Work out the finished part from the listing and answer in its coordinate system (mm). Face numbers are marked on the shaded views. A direction names the side the tool comes from. Round coordinates to 2 decimals unless told otherwise and drop trailing zeros. Loops run counter-clockwise (first coordinate to the right, second up) from the corner with the lowest first, then second, coordinate; pieces in that order, holes last. Notation, with made-up numbers: (-5.5, 17) -> (4.5, 17) arc R25 ccw to (4.5, 49) -> close; hole circle Ø1 at (25, 83). An arc over 180 degrees is marked (long way). Use one line per item in the form item = value.
```python
from build123d import *

# Parameters (mm, degrees)
F1_DEPTH = 63.5
F0_W     = 25.4
F0_H     = 19.05
F2_DEPTH = 25.4
F3_DEPTH = 7.9375
F4_DEPTH = 25.4
F5_DEPTH = 63.5
F7_R     = 6.35


with BuildPart() as f1:
    # F0 (on Front) → F1 (new body)
    with BuildSketch(Plane.XZ):
        Polygon((-41.275, 9.525), (-41.275, -9.525), (41.275, -9.525), (41.275, 9.525), (22.225, 9.525), align=None)
    extrude(amount=F1_DEPTH)

    # F0 (on Front) → F2 (join)
    with BuildSketch(Plane.XZ):
        with Locations((73.025, 52.4002)):
            Rectangle(F0_W, F0_H)
        with BuildLine():
            Line((22.225, 9.525), (41.275, 9.525))
            Line((41.275, 9.525), (41.275, 27.0002))
            ThreePointArc((41.275, 27.0002), (45.9246798487, 38.2255201513), (57.15, 42.8752))
            Line((57.15, 42.8752), (60.325, 42.8752))
            Line((60.325, 42.8752), (60.325, 61.9252))
            Line((60.325, 61.9252), (57.15, 61.9252))
            add(Edge.make_bspline(
                [(52.9823235554, 61.6756394068), (54.3561666256, 61.7778957216), (55.7451531138, 61.8610815688), (57.15, 61.9252)],
                knots=[107.6072789541, 107.6072789541, 107.6072789541, 107.6072789541, 111.5045361635, 111.5045361635, 111.5045361635, 111.5045361635], degree=3))
            ThreePointArc((52.9823235554, 61.6756394068), (31.0223161682, 50.1756128892), (22.225, 27.0002))
            Line((22.225, 27.0002), (22.225, 9.525))
        make_face()
    extrude(amount=F2_DEPTH)

    # F0 (on Front) → F3 (join, symmetric)
    with BuildSketch(Plane.XZ):
        with BuildLine():
            add(Edge.make_bspline(
                [(-41.275, 9.525), (-11.3392454838, 41.4901042483), (15.0491037151, 58.8522374069), (52.9823235554, 61.6756394068)],
                knots=[0, 0, 0, 0, 107.6072789541, 107.6072789541, 107.6072789541, 107.6072789541], degree=3))
            Line((-41.275, 9.525), (22.225, 9.525))
            Line((22.225, 9.525), (22.225, 27.0002))
            ThreePointArc((22.225, 27.0002), (31.0223161682, 50.1756128892), (52.9823235554, 61.6756394068))
        make_face()
    extrude(amount=F3_DEPTH, both=True)

    # F0 (on Front) → F4 (join, symmetric)
    with BuildSketch(Plane.XZ):
        with BuildLine():
            Line((22.225, 9.525), (41.275, 9.525))
            Line((41.275, 9.525), (41.275, 27.0002))
            ThreePointArc((41.275, 27.0002), (45.9246798487, 38.2255201513), (57.15, 42.8752))
            Line((57.15, 42.8752), (60.325, 42.8752))
            Line((60.325, 42.8752), (60.325, 61.9252))
            Line((60.325, 61.9252), (57.15, 61.9252))
            add(Edge.make_bspline(
                [(52.9823235554, 61.6756394068), (54.3561666256, 61.7778957216), (55.7451531138, 61.8610815688), (57.15, 61.9252)],
                knots=[107.6072789541, 107.6072789541, 107.6072789541, 107.6072789541, 111.5045361635, 111.5045361635, 111.5045361635, 111.5045361635], degree=3))
            ThreePointArc((52.9823235554, 61.6756394068), (31.0223161682, 50.1756128892), (22.225, 27.0002))
            Line((22.225, 27.0002), (22.225, 9.525))
        make_face()
        with Locations((73.025, 52.4002)):
            Rectangle(F0_W, F0_H)
    extrude(amount=F4_DEPTH, both=True)

    # F0 (on Front) → F5 (join)
    with BuildSketch(Plane.XZ):
        Polygon((-41.275, 9.525), (-41.275, -9.525), (41.275, -9.525), (41.275, 9.525), (22.225, 9.525), align=None)
    extrude(amount=-F5_DEPTH)

    # F0 (on Front) → F6 (revolve)
    with BuildSketch(Plane.XZ):
        Polygon((85.725, 66.675), (85.725, 61.9252), (85.725, 42.8752), (85.725, 38.1), (111.125, 38.1), (111.125, 66.675), align=None)
    revolve(axis=Axis((85.725, 0, 52.3875), (0, 0, 1)))

    # F7
    f7_edges = [f1.edges().sort_by_distance(p)[0] for p in [
        (-41.275, -63.5, 0),
        (41.275, -63.5, 0),
        (41.275, 63.5, 0),
        (-41.275, 63.5, 0),
    ]]
    fillet(f7_edges, radius=F7_R)


solid = f1.part
```
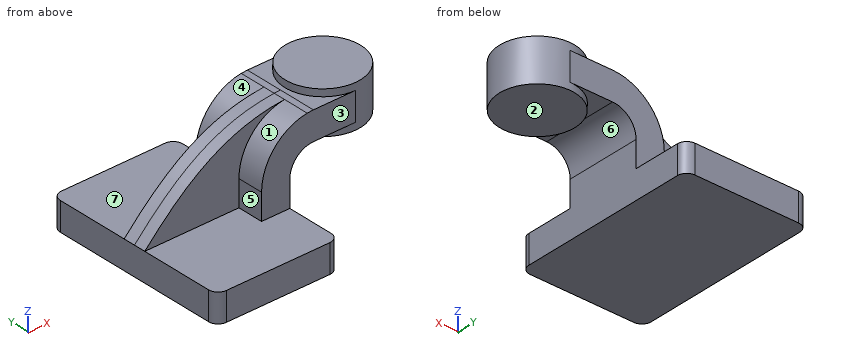
(1) Find section A-A, the plane z = 5. Write down the section's boundary in (x, y) (3 decimals), then the cut area to 3 significant figures.
Completed:
outline = (-41.275, -57.15) arc R6.35 ccw to (-34.925, -63.5) -> (34.925, -63.5) arc R6.35 ccw to (41.275, -57.15) -> (41.275, 57.15) arc R6.35 ccw to (34.925, 63.5) -> (-34.925, 63.5) arc R6.35 ccw to (-41.275, 57.15) -> close
area = 10,400 mm2
(2) Find section B-B, the plane y = -28. Write down the section's boundary in (x, z) (3 decimals).
Completed:
outline = (-41.275, -9.525) -> (41.275, -9.525) -> (41.275, 9.525) -> (-41.275, 9.525) -> close
(3) Find section C-C, the plane x = 91.5. Write down the section's boundary in (y, z) (3 decimals).
Completed:
outline = (-24.735, 38.1) -> (24.735, 38.1) -> (24.735, 66.675) -> (-24.735, 66.675) -> close
(4) For the marked faces 1, 2, 3 and 4, determine the directions among +Z, -Z, +X, -X, +Y, -Y from which every point of the face is accessible in a straight line to the end or side of a thin tool.
Completed:
face_1 = +Z, -X, -Y
face_2 = -Z, +X, +Y, -Y
face_3 = +Z, +X, -X, -Y
face_4 = +Z, -X, +Y
(5) Given P1, Ø8.5, axis at y = -14, z = 21, coming from the -X side (3 decimals); P2, Ø12, axis at y = 42.5, z = 9, coming from the +X side (3 decimals); P3, Ø12, axis at x = 78.5, z = 54.5, coming from the -Y side; P4, Ø8, axis at x = 0, z = 51, coming from the +Y side, each flat-ended and moving along its own axis, determine where each tip first touches the part or whether it passes through.
Completed:
P1 = 22.225
P2 = 41.275
P3 = -25.4
P4 = through
(6) For a pull along X with two mould halves and no side action, classify the marked faces 5, 6 and 7 as +X half, -X half, draft (parallel to the pull), parting line (faces both ways), or undercut.
Completed:
face_5 = -X half
face_6 = undercut
face_7 = draft
(7) Consider L1, parallel to X at y = -13.5, z = 26.5 (3 decimals); L2, parallel to Z at x = 11.5, y = 57.5 (3 decimals); L3, parallel to Y at x = 14, z = 21. Determine where each line is inside the solid, lowest interval first.
Completed:
L1 = 22.225 to 41.275
L2 = -9.525 to 9.525
L3 = -7.94 to 7.94
